Read the model definition and answer for the solid it produces. Units are mm, in the model's axes. Face numbers are marked on the shaded views. A direction names the side the tool comes from. Give positions to 0.01 mm unless a question says otherwise; leave off trailing zeros. Write each loop counter-clockwise with the first axis right and the second up, starting at its lowest first coordinate (ties: lowest second). Pieces come first, ordered by that corner, then holes. Notation, with made-up numbers: (11, 81.25) - (36, 81.25) arc R18 ccw to (36, 100.25) - close; hole circle Ø9 at (84.25, 68). An arc over 180 degrees is marked (long way). Answer as a JSON object with one key per item and string values. Group by question number.
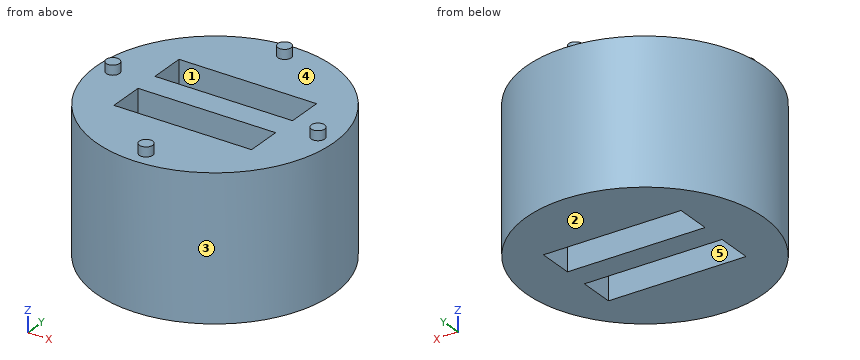
```python
from build123d import *

# Parameters (mm, degrees)
F0_R     = 15.875
F1_DEPTH = 19.05
F6_W     = 18.382654
F6_H     = 4.7625
F7_DEPTH = 19.05
F3_R     = 0.889
F8_DEPTH = 20.32


with BuildPart() as f1:
    # F0 (on Top) → F1 (new body)
    with BuildSketch(Plane.XY):
        Circle(F0_R)
    extrude(amount=F1_DEPTH)

    # F6 (on face) → F7 (cut)
    with BuildSketch(Plane.XY.offset(19.05)):
        with Locations((0.03649, 4.055353)):
            Rectangle(F6_W, F6_H)
        with Locations((0.03649, -4.055353)):
            Rectangle(F6_W, F6_H)
    extrude(amount=-F7_DEPTH, mode=Mode.SUBTRACT)

    # F3 (on face) → F8 (join)
    with BuildSketch(Plane(origin=(0, 0, 0), x_dir=(1, 0, 0), z_dir=(0, 0, -1))):
        with Locations((0, 13.652203)):
            Circle(F3_R)
        with Locations((-13.659894, -0.015021)):
            Circle(F3_R)
        with Locations((0.062219, -13.682245)):
            Circle(F3_R)
        with Locations((13.674476, -0.124876)):
            Circle(F3_R)
    extrude(amount=-F8_DEPTH)


solid = f1.part
```
1) Which of the six approach directions +Z, -Z, +X, -X, +Y, -Y give full straight-line access (tool end or side, diameter ignored) to the marked faces 4 and 5?
2) Find section B-B, the plane x = 0. Write down the section's boundary in (y, z) (3 decimals), and give its area (3 significant figures).
3) Flat-ended cylindrical pins translate along their axes: pin 1 Ø4 at (y, z) = (-6.5, 14) entering from +X; pin 2 Ø4 at (x, z) = (-7, 17.5) entering from +Y; pin 3 Ø5 at (y, z) = (5.5, 9.5) entering from +X. Find the tip coordinate at first contact, or state that the pin passes through.
4) Find section A-A, the plane z = 17. Write down the section's boundary in (x, y) (3 decimals).
5) Find the intervals of material crossed by line 1 (Y direction, x = 0, z = 15.5) (3 decimals); line 2 (Y direction, x = 5, z = 3.5); line 3 (Z direction, x = 9.5, y = 11.5), in increasing order. Write a range as [from, to].
6) For a pull along Y with two mould halves and no side action, classify the marked faces 1, 2 and 3 as released by +Y, released by -Y, zero draft, split by the parting line, or undercut.
7) Find section C-C, the plane x = 6. Write down the section's boundary in (y, z).
8) Find section D-D, the plane y = 10. Write down the section's boundary in (x, z), and give its area (3 significant figures).
Values follow:
{
 "1": {"face 4": "+Z", "face 5": "+Z, -Z"},
 "2": {"outline": "(-15.875, 0) - (-6.437, 0) - (-6.437, 19.05) - (-12.763, 19.05) - (-12.763, 20.32) - (-14.541, 20.32) - (-14.541, 19.05) - (-15.875, 19.05) - close; (-1.674, 0) - (1.674, 0) - (1.674, 19.05) - (-1.674, 19.05) - close; (6.437, 0) - (15.875, 0) - (15.875, 19.05) - (14.569, 19.05) - (14.569, 20.32) - (12.795, 20.32) - (12.795, 19.05) - (6.437, 19.05) - close", "area": "428 mm2"},
 "3": {"pin 1": "stops at x = 15.22", "pin 2": "stops at y = 15.07", "pin 3": "stops at x = 15.59"},
 "4": {"outline": "circle Ø31.75 at (0, 0); hole (-9.155, -6.437) - (9.228, -6.437) - (9.228, -1.674) - (-9.155, -1.674) - close; hole (-9.155, 1.674) - (9.228, 1.674) - (9.228, 6.437) - (-9.155, 6.437) - close"},
 "5": {"line 1": "y = [-15.875, -6.437], [-1.674, 1.674], [6.437, 15.875]", "line 2": "y = [-15.07, -6.44], [-1.67, 1.67], [6.44, 15.07]", "line 3": "z = [0, 19.05]"},
 "6": {"face 1": "undercut", "face 2": "zero draft", "face 3": "split by the parting line"},
 "7": {"outline": "(-14.7, 0) - (-6.44, 0) - (-6.44, 19.05) - (-14.7, 19.05) - close; (-1.67, 0) - (1.67, 0) - (1.67, 19.05) - (-1.67, 19.05) - close; (6.44, 0) - (14.7, 0) - (14.7, 19.05) - (6.44, 19.05) - close"},
 "8": {"outline": "(-12.33, 0) - (12.33, 0) - (12.33, 19.05) - (-12.33, 19.05) - close", "area": "470 mm2"}
}
